CAD build for the part. Positions are in the model's coordinates, mm. Face numbers are marked on the shaded views. Coordinates: 2 decimals unless noted, no trailing zeros. Write each loop counter-clockwise with the first axis right and the second up, starting at its lowest first coordinate (ties: lowest second). Pieces come first, ordered by that corner, then holes.
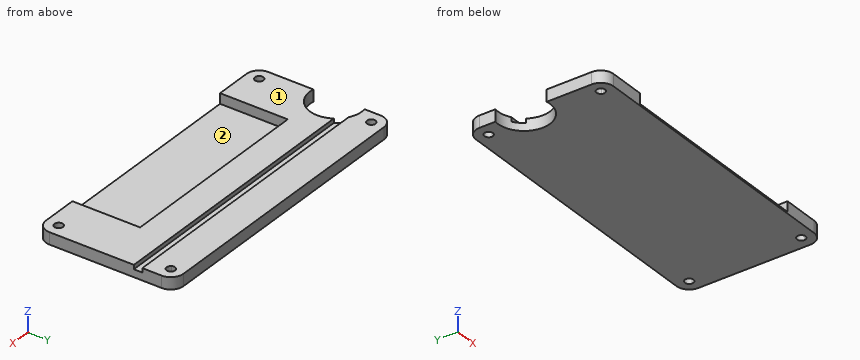
```python
from build123d import *

# Parameters (mm, degrees)
F1_DEPTH = 2.8
F2_W     = 48
F2_H     = 2
F2_H_2   = 16
F3_DEPTH = 2.4
F4_DEPTH = 1


with BuildPart() as f1:
    # F0 (on Top) → F1 (new body)
    with BuildSketch(Plane.XY):
        with BuildLine():
            ThreePointArc((34.8248369992, 13.6349746287), (33.9461573427, 15.7562949722), (31.8248369992, 16.6349746287))
            Line((31.8248369992, 16.6349746287), (-33.3311557472, 16.6349746287))
            ThreePointArc((-33.3311557472, 16.6349746287), (-35.4524760907, 15.7562949722), (-36.3311557472, 13.6349746287))
            Line((-36.3311557472, 13.6349746287), (-36.3311557472, 9.882260114))
            ThreePointArc((-36.3311557472, 9.882260114), (-29.2342316353, 3.8106893189), (-36.3311557472, -2.2608814761))
            Line((-36.3311557472, -2.2608814761), (-36.3311557472, -12.8735043705))
            ThreePointArc((-36.3311557472, -12.8735043705), (-35.4524760907, -14.994824714), (-33.3311557472, -15.8735043705))
            Line((-33.3311557472, -15.8735043705), (31.8248369992, -15.8735043705))
            ThreePointArc((31.8248369992, -15.8735043705), (33.9461573427, -14.994824714), (34.8248369992, -12.8735043705))
            Line((34.8248369992, -12.8735043705), (34.8248369992, 13.6349746287))
        make_face()
        with BuildLine():
            ThreePointArc((-32.3311557472, -12.8735043705), (-34.3042365532, -13.1039685651), (-32.4373832372, -12.4249838019))
            ThreePointArc((-32.4373832372, -12.4249838019), (-32.3580749412, -12.6430401758), (-32.3311557472, -12.8735043705))
        make_face(mode=Mode.SUBTRACT)
        with BuildLine():
            ThreePointArc((32.8248369992, -12.8735043705), (31.5943728046, -13.8465851764), (30.9310644892, -12.4249838019))
            ThreePointArc((30.9310644892, -12.4249838019), (32.0553011938, -11.9004235645), (32.8248369992, -12.8735043705))
        make_face(mode=Mode.SUBTRACT)
        with BuildLine():
            ThreePointArc((-32.3311557472, 13.6349746287), (-32.3580749412, 13.4045104341), (-32.4373832372, 13.1864540602))
            ThreePointArc((-32.4373832372, 13.1864540602), (-34.3042365532, 13.8654388233), (-32.3311557472, 13.6349746287))
        make_face(mode=Mode.SUBTRACT)
        with BuildLine():
            ThreePointArc((32.8248369992, 13.6349746287), (32.0553011938, 12.6618938227), (30.9310644892, 13.1864540602))
            ThreePointArc((30.9310644892, 13.1864540602), (31.5943728046, 14.6080554347), (32.8248369992, 13.6349746287))
        make_face(mode=Mode.SUBTRACT)
    extrude(amount=F1_DEPTH)

    # F2 (on face) → F3 (cut)
    with BuildSketch(Plane.XY.offset(2.8)):
        with Locations((-0.753159374, -16.8735043705)):
            Rectangle(F2_W, F2_H)
        with Locations((-0.753159374, -7.8735043705)):
            Rectangle(F2_W, F2_H_2)
    extrude(amount=-F3_DEPTH, mode=Mode.SUBTRACT)

    # F2 (on face) → F4 (cut)
    with BuildSketch(Plane.XY.offset(2.8)):
        with BuildLine():
            Line((-30.1732155819, 7.075597696), (34.8248369992, 7.075597696))
            Line((34.8248369992, 7.075597696), (34.8248369992, 9.075597696))
            Line((34.8248369992, 9.075597696), (-32.2097548914, 9.075597696))
            ThreePointArc((-32.2097548914, 9.075597696), (-31.0737619928, 8.1954717029), (-30.1732155819, 7.075597696))
        make_face()
    extrude(amount=-F4_DEPTH, mode=Mode.SUBTRACT)


solid = f1.part
```
Item 1: Saw through at A-A, the plane z = 2.35. Write the cut outline in (x, y), and give its area (3 significant figures).
Item 2: Saw through at C-C, the plane x = -19.5. Write the cut outline in (y, z).
Item 3: Saw through at D-D, the plane y = 2. Write the cut outline in (x, z).
Item 4: Flat gauge pins, fed straight in: pin 1 Ø1.6 at (x, y) = (-33.33, 13.63) entering from -Z; pin 2 Ø1.2 at (x, z) = (-2.5, 2) entering from -Y. Where does each tip first touch, or does it go through?
Item 5: Wall check: line 1 along Y through (x, z) = (32, 0.75); line 2 along Y through (x, z) = (22, 2.05); line 3 along X through (y, z) = (-10, 1.8). Give the ranges that are in metal, low to high.
Item 6: Two-plate mould, pull along X, no slides. Class the marked faces 1 and 2: +X half, -X half, draft (parallel to the pull), parting line (faces both ways), or undercut.
Item 7: Saw through at B-B, the plane y = -5. Write the cut outline in (x, z), and give its area (3 significant figures).
Working result:
1. outline: (-36.33, -12.87) arc R3 ccw to (-33.33, -15.87) - (-24.75, -15.87) - (-24.75, 0.13) - (23.25, 0.13) - (23.25, -15.87) - (31.82, -15.87) arc R3 ccw to (34.82, -12.87) - (34.82, 7.08) - (-30.17, 7.08) arc R6.15 cw to (-36.33, -2.26) - close; (-36.33, 9.88) arc R6.15 cw to (-32.21, 9.08) - (34.82, 9.08) - (34.82, 13.63) arc R3 ccw to (31.82, 16.63) - (-33.33, 16.63) arc R3 ccw to (-36.33, 13.63) - close; hole circle Ø2 at (-33.33, -12.87); hole circle Ø2 at (-33.33, 13.63); hole circle Ø2 at (31.82, -12.87); hole circle Ø2 at (31.82, 13.63)
1. area: 1,320 mm2
2. outline: (-15.87, 0) - (16.63, 0) - (16.63, 2.8) - (9.08, 2.8) - (9.08, 1.8) - (7.08, 1.8) - (7.08, 2.8) - (0.13, 2.8) - (0.13, 0.4) - (-15.87, 0.4) - close
3. outline: (-29.51, 0) - (34.82, 0) - (34.82, 2.8) - (-29.51, 2.8) - close
4. pin 1: passes through
4. pin 2: stops at y = 0.13
5. line 1: y = -15.87 to -13.86, -11.89 to 12.65, 14.62 to 16.63
5. line 2: y = 0.13 to 7.08, 9.08 to 16.63
5. line 3: x = -36.33 to -24.75, 23.25 to 34.82
6. face 1: draft
6. face 2: undercut
7. outline: (-36.33, 0) - (34.82, 0) - (34.82, 2.8) - (23.25, 2.8) - (23.25, 0.4) - (-24.75, 0.4) - (-24.75, 2.8) - (-36.33, 2.8) - close
7. area: 84.0 mm2
